```python
from build123d import *

# Parameters (mm, degrees)
F0_R     = 9.4
F1_DEPTH = 3


with BuildPart() as f1:
    # F0 (on Front) → F1 (new body)
    with BuildSketch(Plane.XZ):
        with BuildLine():
            Line((58.8, 11.4), (0, 11.4))
            ThreePointArc((0, 11.4), (-9.870808, 5.703258), (-9.87645, -5.693483))
            Line((-9.87645, -5.693483), (-0.07645, -22.693483))
            Line((-0.07645, -22.693483), (19.523115, -56.692727))
            Line((19.523115, -56.692727), (29.322897, -73.692349))
            ThreePointArc((29.322897, -73.692349), (33.496089, -77.869674), (39.199347, -79.398866))
            Line((39.199347, -79.398866), (41.449014, -79.398866))
            ThreePointArc((41.449014, -79.398866), (48.999129, -75.598489), (56.549243, -79.398866))
            Line((56.549243, -79.398866), (61.049014, -79.398866))
            ThreePointArc((61.049014, -79.398866), (68.599129, -75.598489), (76.149243, -79.398866))
            Line((76.149243, -79.398866), (80.649014, -79.398866))
            ThreePointArc((80.649014, -79.398866), (88.199129, -75.598489), (95.749243, -79.398866))
            Line((95.749243, -79.398866), (100.249014, -79.398866))
            ThreePointArc((100.249014, -79.398866), (107.799129, -75.598489), (115.349243, -79.398866))
            Line((115.349243, -79.398866), (119.849014, -79.398866))
            ThreePointArc((119.849014, -79.398866), (127.399129, -75.598489), (134.949243, -79.398866))
            Line((134.949243, -79.398866), (139.449014, -79.398866))
            ThreePointArc((139.449014, -79.398866), (146.999129, -75.598489), (154.549243, -79.398866))
            Line((154.549243, -79.398866), (156.799347, -79.398866))
            ThreePointArc((156.799347, -79.398866), (158.034478, -79.331759), (159.255068, -79.131226))
            ThreePointArc((159.255068, -79.131226), (161.904503, -76.85475), (165.20223, -75.702862))
            ThreePointArc((165.20223, -75.702862), (170.133763, -76.288359), (174.078718, -79.305006))
            Line((174.078718, -79.305006), (176.475578, -79.305006))
            Line((176.475578, -79.305006), (166.675796, -62.305384))
            Line((166.675796, -62.305384), (127.47645, 5.693483))
            ThreePointArc((127.47645, 5.693483), (123.303258, 9.870808), (117.6, 11.4))
            Line((117.6, 11.4), (98, 11.4))
            Line((98, 11.4), (58.8, 11.4))
        make_face()
        with Locations((39.199347, -67.998866)):
            Circle(F0_R, mode=Mode.SUBTRACT)
        with Locations((58.799347, -67.998866)):
            Circle(F0_R, mode=Mode.SUBTRACT)
        with Locations((78.399347, -67.998866)):
            Circle(F0_R, mode=Mode.SUBTRACT)
        with Locations((29.399564, -50.999244)):
            Circle(F0_R, mode=Mode.SUBTRACT)
        with Locations((19.599782, -33.999622)):
            Circle(F0_R, mode=Mode.SUBTRACT)
        with Locations((48.999564, -50.999244)):
            Circle(F0_R, mode=Mode.SUBTRACT)
        with Locations((68.599564, -50.999244)):
            Circle(F0_R, mode=Mode.SUBTRACT)
        with Locations((39.199782, -33.999622)):
            Circle(F0_R, mode=Mode.SUBTRACT)
        with Locations((58.799782, -33.999622)):
            Circle(F0_R, mode=Mode.SUBTRACT)
        with Locations((78.399782, -33.999622)):
            Circle(F0_R, mode=Mode.SUBTRACT)
        with Locations((97.999347, -67.998866)):
            Circle(F0_R, mode=Mode.SUBTRACT)
        with Locations((117.599347, -67.998866)):
            Circle(F0_R, mode=Mode.SUBTRACT)
        with Locations((137.199347, -67.998866)):
            Circle(F0_R, mode=Mode.SUBTRACT)
        with Locations((156.799347, -67.998866)):
            Circle(F0_R, mode=Mode.SUBTRACT)
        with Locations((88.199564, -50.999244)):
            Circle(F0_R, mode=Mode.SUBTRACT)
        with Locations((107.799564, -50.999244)):
            Circle(F0_R, mode=Mode.SUBTRACT)
        with Locations((127.399564, -50.999244)):
            Circle(F0_R, mode=Mode.SUBTRACT)
        with Locations((97.999782, -33.999622)):
            Circle(F0_R, mode=Mode.SUBTRACT)
        with Locations((117.599782, -33.999622)):
            Circle(F0_R, mode=Mode.SUBTRACT)
        with Locations((146.999564, -50.999244)):
            Circle(F0_R, mode=Mode.SUBTRACT)
        with Locations((137.199782, -33.999622)):
            Circle(F0_R, mode=Mode.SUBTRACT)
        with BuildLine():
            ThreePointArc((9.8, -26.4), (5.097314, -25.139087), (1.656261, -21.694626))
            ThreePointArc((1.656261, -21.694626), (7.370097, -7.919495), (19.2, -17))
            ThreePointArc((19.2, -17), (16.446804, -23.646804), (9.8, -26.4))
        make_face(mode=Mode.SUBTRACT)
        with Locations((29.4, -17)):
            Circle(F0_R, mode=Mode.SUBTRACT)
        with Locations((49, -17)):
            Circle(F0_R, mode=Mode.SUBTRACT)
        with BuildLine():
            ThreePointArc((76.743739, -12.305374), (77.680505, -14.570097), (78, -17))
            ThreePointArc((78, -17), (75.246804, -23.646804), (68.6, -26.4))
            ThreePointArc((68.6, -26.4), (60.460913, -12.297314), (76.743739, -12.305374))
        make_face(mode=Mode.SUBTRACT)
        with BuildLine():
            ThreePointArc((0, 9.4), (6.646804, 6.646804), (9.4, 0))
            ThreePointArc((9.4, 0), (2.429903, -9.080505), (-8.143739, -4.694626))
            ThreePointArc((-8.143739, -4.694626), (-8.139087, 4.702686), (0, 9.4))
        make_face(mode=Mode.SUBTRACT)
        with BuildLine():
            ThreePointArc((29, 0), (12.953196, -6.646804), (19.6, 9.4))
            ThreePointArc((19.6, 9.4), (26.246804, 6.646804), (29, 0))
        make_face(mode=Mode.SUBTRACT)
        with BuildLine():
            ThreePointArc((48.6, 0), (32.553196, -6.646804), (39.2, 9.4))
            ThreePointArc((39.2, 9.4), (45.846804, 6.646804), (48.6, 0))
        make_face(mode=Mode.SUBTRACT)
        with BuildLine():
            ThreePointArc((68.2, 0), (52.153196, -6.646804), (58.8, 9.4))
            ThreePointArc((58.8, 9.4), (63.502686, 8.139087), (66.943739, 4.694626))
            ThreePointArc((66.943739, 4.694626), (67.880505, 2.429903), (68.2, 0))
        make_face(mode=Mode.SUBTRACT)
        with Locations((78.4, 0)):
            Circle(F0_R, mode=Mode.SUBTRACT)
        with Locations((88.2, -17)):
            Circle(F0_R, mode=Mode.SUBTRACT)
        with Locations((107.8, -17)):
            Circle(F0_R, mode=Mode.SUBTRACT)
        with Locations((127.4, -17)):
            Circle(F0_R, mode=Mode.SUBTRACT)
        with Locations((98, 0)):
            Circle(F0_R, mode=Mode.SUBTRACT)
        with Locations((117.6, 0)):
            Circle(F0_R, mode=Mode.SUBTRACT)
    extrude(amount=F1_DEPTH)


solid = f1.part
```
Here's how the part is built. I have some questions about the finished solid (model axes, mm). Round coordinates to 2 decimals unless told otherwise and drop trailing zeros. Order: outer loops, then holes, each group sorted by start corner. A loop starts at its lowest first (then second) coordinate and runs counter-clockwise, first axis right, second up. Notation, with made-up numbers: M 60.25,49 L 116.25,49 A32 cw 116.25,83 Z; hole C -38,41 d6. An arc over 180 degrees is marked long. Answer in a Markdown table with one row per item.
Item 1: Imagine slicing it at A-A, the plane z = -20. State how many separate pieces and enclosed holes the cut face has, and give its area (3 significant figures).
A:
| item | result |
|---|---|
| separate pieces | 8 |
| enclosed holes | 0 |
| area | 57.6 mm2 |
Item 2: I'm going to push a flat-ended pin straight in: pin 1 (1 mm diameter, centred on x = 147, y = -2, fed in from -Z). Where does the tip first touch, or does it pass through?
A:
| item | result |
|---|---|
| pin 1 | stops at z = -75.61 |
Item 3: Imagine slicing it at B-B, the plane x = 161. Write out the boundary of the cut face in (y, z), and give its area (3 significant figures).
A:
| item | result |
|---|---|
| outline | M -3,-77.45 L 0,-77.45 L 0,-76.41 L -3,-76.41 Z; M -3,-59.59 L 0,-59.59 L 0,-52.46 L -3,-52.46 Z |
| area | 24.5 mm2 |
Item 4: Thinking about a two-plate mould opening in X: for faces 1 (the face through (68, -3, -27)), 2 (the face through (78.81, -1.48, -16.59)), 3 (the face through (-9.786, -1.479, 5.847)), which applies, +X half, -X half, draft (parallel to the pull), parting line (faces both ways), or undercut?
A:
| item | result |
|---|---|
| face 1 | draft |
| face 2 | undercut |
| face 3 | -X half |
Item 5: If I drill on L1, parallel to Z at x = 21.5, y = -2.15; L2, parallel to Z at x = 130, y = -1.3; L3, parallel to Z at x = 142.5, y = -2, over which ranges is the centre line in solid material (lowest first)? Write a range as from..to.
A:
| item | result |
|---|---|
| L1 | z = -60.12..-56.09, -45.9..-43.21, -24.79..-22.09, -11.91..-9.21, 9.21..11.4 |
| L2 | z = -75.97..-74.04, -61.95..-60.03, -41.97..-40.04, -27.96..-26.03, -7.97..1.32 |
| L3 | z = -76.75..-75.76, -60.24..-59.25, -42.75..-41.76, -26.24..-20.37 |
